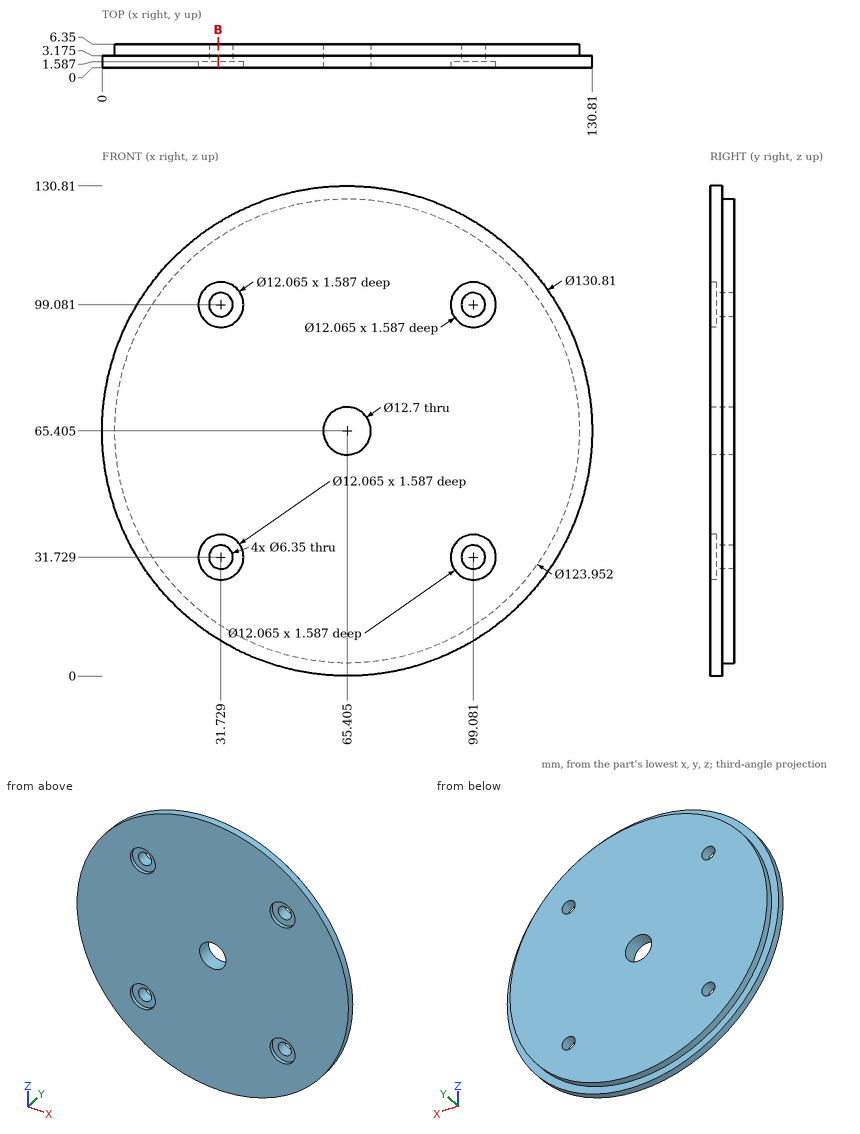
The figure shows three views and two pictorial views of one solid part (mm, origin at its lowest corner). Answer the questions. Coordinates: 2 decimals unless noted, no trailing zeros. Answer as a JSON object with one key per item and string values.
Q1. Flat-ended cylindrical pins translate along their axes: pin 1 Ø4 at (x, z) = (31.73, 99.08) entering from -Y; pin 2 Ø1 at (y, z) = (3.5, 96) entering from +X; pin 3 Ø9.5 at (x, z) = (31.73, 31.73) entering from -Y; pin 4 Ø1 at (x, y) = (29, 5.5) entering from +Z. Find the tip coordinate at first contact, or state that the pin passes through.
The answers:
{"pin 1": "passes through", "pin 2": "stops at x = 123.41", "pin 3": "stops at y = 1.59", "pin 4": "stops at z = 115.92"}
Q2. The part is cut by section B-B on x = 31. Give the number of separate pieces and of enclosed holes in the cut face.
The answers:
{"separate pieces": "3", "enclosed holes": "0"}
Q3. Consider line 1 (Y direction, x = 113, z = 107.5) (1 decimal); line 2 (X direction, y = 3.75, z = 67); line 3 (X direction, y = 5, z = 48). Determine where each line is inside the solid, lowest interval first. Write a range as [from, to].
The answers:
{"line 1": "y = [0, 3.2]", "line 2": "x = [3.45, 59.26], [71.55, 127.36]", "line 3": "x = [5.92, 124.89]"}
